The listing builds one solid part. Answer for the finished solid, in the listing's coordinates (mm). Face numbers are marked on the shaded views. A direction names the side the tool comes from. Round coordinates to 2 decimals unless told otherwise and drop trailing zeros. Loops run counter-clockwise (first coordinate to the right, second up) from the corner with the lowest first, then second, coordinate; pieces in that order, holes last. Notation, with made-up numbers: (-31, 2.25) -> (12, 2.25) arc R18 ccw to (12, 30.25) -> close; hole circle Ø11 at (-25.5, 60.5). An arc over 180 degrees is marked (long way). One line per question, with ' | ' between items.
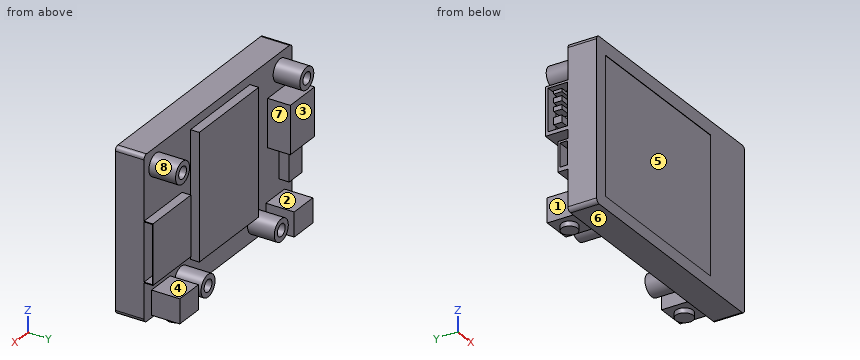
from build123d import *

# Parameters (mm, degrees)
ESBO_O1_W                = 57.2
ESBO_O1_H                = 40
RESSALTO_EXTRUS_O1_DEPTH = 7.1
ESBO_O2_R                = 2.7
RESSALTO_EXTRUS_O2_DEPTH = 6.6
ESBO_O3_R                = 1.5
CORTE_EXTRUS_O1_DEPTH    = 6.6
ESBO_O4_W                = 40.649985971
ESBO_O4_H                = 33.681416947
CORTE_EXTRUS_O2_DEPTH    = 0.1
ESBO_O5_W                = 14.7
ESBO_O5_H                = 14.7
RESSALTO_EXTRUS_O3_DEPTH = 2.2
ESBO_O6_W                = 14.368584986
ESBO_O6_H                = 2.042443489
CORTE_EXTRUS_O3_DEPTH    = 10
ESBO_O7_W                = 9.4
ESBO_O7_H                = 11.8
ESBO_O7_W_2              = 5
ESBO_O7_H_2              = 7.3
RESSALTO_EXTRUS_O4_DEPTH = 2.5
ESBO_O8_W                = 9.4
ESBO_O8_H                = 11.8
RESSALTO_EXTRUS_O5_DEPTH = 3.1
ESBO_O9_W                = 5.766531476
ESBO_O9_H                = 1.868031324
ESBO_O9_W_2              = 10.396000408
ESBO_O9_H_2              = 4.791906438
ESBO_O9_W_3              = 1.746203194
ESBO_O9_H_3              = 2.030468829
ESBO_O9_W_4              = 1.096453168
ESBO_O9_W_5              = 1.218281297
ESBO_O9_W_6              = 0.771578155
CORTE_EXTRUS_O4_DEPTH    = 3.1
FILETE1_R                = 1
ESBO_O10_W               = 22.938206369
ESBO_O10_H               = 30.952060747
RESSALTO_EXTRUS_O6_DEPTH = 2.2
ESBO_O11_W               = 7.2
ESBO_O11_H               = 6
RESSALTO_EXTRUS_O7_DEPTH = 7
ESBO_O12_R               = 2.135826149
ESBO_O12_R_2             = 1.975311567
RESSALTO_EXTRUS_O8_DEPTH = 1.2


with BuildPart() as part:
    # Esboço1 → Ressalto-extrusão1 (new body)
    with BuildSketch(Plane(origin=(0, 0, 0), x_dir=(1, 0, 0), z_dir=(0, 1, 0))):
        with Locations((28.6, 20)):
            Rectangle(ESBO_O1_W, ESBO_O1_H)
    extrude(amount=RESSALTO_EXTRUS_O1_DEPTH)

    # Esboço2 → Ressalto-extrusão2 (add)
    with BuildSketch(Plane(origin=(0, 7.1, 0), x_dir=(1, 0, 0), z_dir=(0, 1, 0))):
        with Locations((4.6, 4.2)):
            Circle(ESBO_O2_R)
        with Locations((52.6, 4.2)):
            Circle(ESBO_O2_R)
        with Locations((42.75, 35.8)):
            Circle(ESBO_O2_R)
        with Locations((14.45, 35.8)):
            Circle(ESBO_O2_R)
    extrude(amount=RESSALTO_EXTRUS_O2_DEPTH)

    # Esboço3 → Corte-extrusão1 (cut)
    with BuildSketch(Plane(origin=(0, 13.7, 0), x_dir=(1, 0, 0), z_dir=(0, 1, 0))):
        with Locations((14.45, 35.8)):
            Circle(ESBO_O3_R)
        with Locations((42.75, 35.8)):
            Circle(ESBO_O3_R)
        with Locations((52.6, 4.2)):
            Circle(ESBO_O3_R)
        with Locations((4.6, 4.2)):
            Circle(ESBO_O3_R)
    extrude(amount=-CORTE_EXTRUS_O1_DEPTH, mode=Mode.SUBTRACT)

    # Esboço4 → Corte-extrusão2 (cut)
    with BuildSketch(Plane(origin=(0, 0, 0), x_dir=(-1, 0, 0), z_dir=(0, -1, 0))):
        with Locations((-23.751037388, 20.174214226)):
            Rectangle(ESBO_O4_W, ESBO_O4_H)
    extrude(amount=-CORTE_EXTRUS_O2_DEPTH, mode=Mode.SUBTRACT)

    # Esboço5 → Ressalto-extrusão3 (add)
    with BuildSketch(Plane(origin=(0, 7.1, 0), x_dir=(1, 0, 0), z_dir=(0, 1, 0))):
        with Locations((49.85, 22.95)):
            Rectangle(ESBO_O5_W, ESBO_O5_H)
    extrude(amount=RESSALTO_EXTRUS_O3_DEPTH)

    # Esboço6 → Corte-extrusão3 (cut)
    with BuildSketch(Plane(origin=(57.2, 0, 0), x_dir=(0, 0, -1), z_dir=(1, 0, 0))):
        with Locations((22.950407173, 8.128512291)):
            Rectangle(ESBO_O6_W, ESBO_O6_H)
    extrude(amount=-CORTE_EXTRUS_O3_DEPTH, mode=Mode.SUBTRACT)

    # Esboço7 → Ressalto-extrusão4 (add)
    with BuildSketch(Plane(origin=(0, 7.1, 0), x_dir=(1, 0, 0), z_dir=(0, 1, 0))):
        with Locations((4.7, 14.6)):
            Rectangle(ESBO_O7_W, ESBO_O7_H)
        with Locations((2.5, 26.35)):
            Rectangle(ESBO_O7_W_2, ESBO_O7_H_2)
    extrude(amount=RESSALTO_EXTRUS_O4_DEPTH)

    # Esboço8 → Ressalto-extrusão5 (add)
    with BuildSketch(Plane(origin=(0, 9.6, 0), x_dir=(1, 0, 0), z_dir=(0, 1, 0))):
        with Locations((4.7, 14.6)):
            Rectangle(ESBO_O8_W, ESBO_O8_H)
    extrude(amount=RESSALTO_EXTRUS_O5_DEPTH)

    # Esboço9 → Corte-extrusão4 (cut)
    with BuildSketch(Plane.ZY):
        with Locations((-26.071101801, 8.149500051)):
            Rectangle(ESBO_O9_W, ESBO_O9_H)
        with Locations((-14.416210718, 9.611437608)):
            Rectangle(ESBO_O9_W_2, ESBO_O9_H_2)
        with Locations((-17.482218651, 9.611437609)):
            Rectangle(ESBO_O9_W_3, ESBO_O9_H_3, mode=Mode.SUBTRACT)
        with Locations((-14.680171666, 9.611437609)):
            Rectangle(ESBO_O9_W_4, ESBO_O9_H_3, mode=Mode.SUBTRACT)
        with Locations((-12.588788772, 9.611437609)):
            Rectangle(ESBO_O9_W_5, ESBO_O9_H_3, mode=Mode.SUBTRACT)
        with Locations((-10.659843384, 9.611437609)):
            Rectangle(ESBO_O9_W_6, ESBO_O9_H_3, mode=Mode.SUBTRACT)
    extrude(amount=-CORTE_EXTRUS_O4_DEPTH, mode=Mode.SUBTRACT)

    # Filete1
    filete1_edges = [part.edges().sort_by_distance(p)[0] for p in [
        (0, 3.55, -40),
        (57.2, 3.55, -40),
        (57.2, 3.55, 0),
        (0, 3.55, 0),
    ]]
    fillet(filete1_edges, radius=FILETE1_R)

    # Esboço10 → Ressalto-extrusão6 (add)
    with BuildSketch(Plane(origin=(0, 7.1, 0), x_dir=(1, 0, 0), z_dir=(0, 1, 0))):
        with Locations((27.787000281, 17.648107954)):
            Rectangle(ESBO_O10_W, ESBO_O10_H)
    extrude(amount=RESSALTO_EXTRUS_O6_DEPTH)

    # Esboço11 → Ressalto-extrusão7 (add)
    with BuildSketch(Plane(origin=(0, 7.1, 0), x_dir=(1, 0, 0), z_dir=(0, 1, 0))):
        with Locations((6.5, 36.4)):
            Rectangle(ESBO_O11_W, ESBO_O11_H)
        with Locations((50.7, 36.4)):
            Rectangle(ESBO_O11_W, ESBO_O11_H)
    extrude(amount=RESSALTO_EXTRUS_O7_DEPTH)

    # Esboço12 → Ressalto-extrusão8 (add)
    with BuildSketch(Plane(origin=(0, 0, -39.4), x_dir=(-1, 0, 0), z_dir=(0, 0, -1))):
        with Locations((-50.742973547, 10.778272234)):
            Circle(ESBO_O12_R)
        with Locations((-6.357026453, 10.778272234)):
            Circle(ESBO_O12_R_2)
    extrude(amount=RESSALTO_EXTRUS_O8_DEPTH)


solid = part.part
Q1. A cutting plane is placed at C-C on y = 8. Give the number of separate pieces and of enclosed holes in the cut face, plus the area to 3 significant figures.
Numbers:
separate pieces: 10 | enclosed holes: 4 | area: 1,030 mm^2
Q2. A cutting plane is placed at A-A on x = 48. Give the vertices of the cut face in (y, z), plus the area to 3 significant figures.
Numbers:
outline: (0, -40) -> (7.1, -40) -> (7.1, -39.4) -> (14.1, -39.4) -> (14.1, -33.4) -> (7.1, -33.4) -> (7.1, -30.3) -> (9.3, -30.3) -> (9.3, -15.6) -> (7.1, -15.6) -> (7.1, 0) -> (0, 0) -> close; hole (7.11, -30.13) -> (9.15, -30.13) -> (9.15, -15.77) -> (7.11, -15.77) -> close | area: 329 mm^2
Q3. A cutting plane is placed at D-D on y = 3.5. Give the vertices of the cut face in (x, z), plus the area to 3 significant figures.
Numbers:
outline: (0, -39) arc R1 ccw to (1, -40) -> (56.2, -40) arc R1 ccw to (57.2, -39) -> (57.2, -1) arc R1 ccw to (56.2, 0) -> (1, 0) arc R1 ccw to (0, -1) -> close | area: 2,290 mm^2
Q4. For the marked faces 1, 2, 3, 4 and 5, determine the directions among +Z, -Z, +X, -X, +Y, -Y from which every point of the face is accessible in a straight line to the end or side of a thin tool.
Numbers:
face 1: -Z, -X, +Y | face 2: -X, +Y | face 3: +X, -X, +Y | face 4: +X, +Y | face 5: -Y
Q5. Given pin 1 Ø0.6 at (x, z) = (2, -11) entering from -Y; pin 2 Ø5 at (y, z) = (11.5, -35.5) entering from +X; pin 3 Ø3 at (y, z) = (9, -37) entering from -X; pin 4 Ø1.5 at (x, z) = (5, -5) entering from +Y, each flat-ended and moving along its own axis, determine where each tip first touches the part or whether it passes through.
Numbers:
pin 1: y = 0 | pin 2: x = 54.3 | pin 3: x = 2.9 | pin 4: y = 13.7
Q6. Find the intervals of material crossed by line 1 (X direction, y = 10.25, z = -4.2); line 2 (X direction, y = 10.25, z = -35.8); line 3 (Z direction, x = 52.6, y = 11.5), in increasing order. Write a range as from..to.
Numbers:
line 1: 1.9..3.1, 6.1..7.3, 49.9..51.1, 54.1..55.3 | line 2: 2.9..10.1, 11.75..12.95, 15.95..17.15, 40.05..41.25, 44.25..45.45, 47.1..54.3 | line 3: -40.6..-33.4, -6.9..-5.7, -2.7..-1.5
Q7. For a pull along Z with two mould halves and no side action, classify the marked faces 6, 7 and 8 as pulls with the +Z half, pulls with the -Z half, needs draft (parallel to the pull), parting line crosses it, or undercut.
Numbers:
face 6: pulls with the -Z half | face 7: needs draft | face 8: undercut
